from build123d import *

# Parameters (mm, degrees)
BODY_DEPTH         = 10
SKETCH2_W          = 2.5
SKETCH2_H          = 0.2
SKETCH2_W_2        = 4.5
SKETCH2_H_2        = 0.775
CUT_EXTRUDE1_DEPTH = 1.65
SKETCH3_R          = 0.757347034
WIRE_2_DEPTH       = 0.5
WIRE_2_DEPTH_BACK  = 2


with BuildPart() as part:
    # Sketch1 → Body (new body)
    with BuildSketch(Plane.XY):
        with BuildLine():
            Line((0.625, -0.775), (-0.625, -0.775))
            ThreePointArc((-0.625, -0.775), (-0.766421356, -0.716421356), (-0.825, -0.575))
            Line((-0.825, -0.575), (-0.825, 0.575))
            ThreePointArc((-0.825, 0.575), (-0.766421356, 0.716421356), (-0.625, 0.775))
            Line((-0.625, 0.775), (0.625, 0.775))
            ThreePointArc((0.625, 0.775), (0.766421356, 0.716421356), (0.825, 0.575))
            Line((0.825, 0.575), (0.825, -0.575))
            ThreePointArc((0.825, -0.575), (0.766421356, -0.716421356), (0.625, -0.775))
        make_face()
        with BuildLine():
            Line((-0.725, -0.575), (-0.725, 0.575))
            ThreePointArc((-0.725, 0.575), (-0.695710678, 0.645710678), (-0.625, 0.675))
            Line((-0.625, 0.675), (0.625, 0.675))
            ThreePointArc((0.625, 0.675), (0.695710678, 0.645710678), (0.725, 0.575))
            Line((0.725, 0.575), (0.725, -0.575))
            ThreePointArc((0.725, -0.575), (0.695710678, -0.645710678), (0.625, -0.675))
            Line((0.625, -0.675), (-0.625, -0.675))
            ThreePointArc((-0.625, -0.675), (-0.695710678, -0.645710678), (-0.725, -0.575))
        make_face(mode=Mode.SUBTRACT)
    extrude(amount=BODY_DEPTH)

    # Sketch2 → Cut-Extrude1 (cut)
    with BuildSketch(Plane.ZY.offset(0.825)):
        with Locations((2.25, 0.675)):
            Rectangle(SKETCH2_W, SKETCH2_H)
        with Locations((6.75, 0.3875)):
            Rectangle(SKETCH2_W_2, SKETCH2_H_2)
    extrude(amount=-CUT_EXTRUDE1_DEPTH, mode=Mode.SUBTRACT)

    # Sketch3 → Wire 2 (add, two sides)
    with BuildSketch(Plane.XY.offset(10)) as wire_2_sk:
        Circle(SKETCH3_R)
    extrude(amount=WIRE_2_DEPTH)
    extrude(wire_2_sk.sketch, amount=-WIRE_2_DEPTH_BACK)


solid = part.part
For this review, take the finished solid that the model builds, in its own axes (mm). Round coordinates to 2 decimals unless told otherwise and drop trailing zeros. Order: outer loops, then holes, each group sorted by start corner. A loop starts at its lowest first (then second) coordinate and runs counter-clockwise, first axis right, second up. Notation, with made-up numbers: (77, 59.25) -> (134, 59.25) arc R23 ccw to (134, 94.25) -> close; hole circle Ø5 at (-35, -19.75). An arc over 180 degrees is marked (long way). Put each result on its own line as item: value.
Q1. Add section A-A on x = 0. Write out the cut boundary in (y, z) (3 decimals).
Check result:
outline: (-0.775, 0) -> (-0.675, 0) -> (-0.675, 8) -> (0.757, 8) -> (0.757, 9) -> (0.775, 9) -> (0.775, 10) -> (0.757, 10) -> (0.757, 10.5) -> (-0.757, 10.5) -> (-0.757, 10) -> (-0.775, 10) -> close; (0.675, 0) -> (0.775, 0) -> (0.775, 1) -> (0.675, 1) -> close; (0.675, 3.5) -> (0.775, 3.5) -> (0.775, 4.5) -> (0.675, 4.5) -> close
Q2. Mouldability with a two-part tool opening along X and no side actions: class faces 1 (the flat face through (0, 0.775, 9.5)), 2 (the flat face through (0, 0, 8)) as pulls with the +X half, pulls with the -X half, needs draft (parallel to the pull), parting line crosses it, or undercut.
Check result:
face 1: needs draft
face 2: undercut
Q3. Add section D-D on z = 7. Write out the cut boundary in (x, y) (3 decimals), plus the area to 3 significant figures.
Check result:
outline: (-0.825, -0.575) arc R0.2 ccw to (-0.625, -0.775) -> (0.625, -0.775) arc R0.2 ccw to (0.825, -0.575) -> (0.825, 0) -> (0.725, 0) -> (0.725, -0.575) arc R0.1 cw to (0.625, -0.675) -> (-0.625, -0.675) arc R0.1 cw to (-0.725, -0.575) -> (-0.725, 0) -> (-0.825, 0) -> close
area: 0.287 mm2
Q4. For probe 1 along Z at (x, y) = (0.15, -0.2); probe 2 along Y at (x, z) = (0.1, 8.75) (3 decimals); probe 3 along Y at (x, z) = (0.15, 8.25) (3 decimals), list the stretches that pass through material, from the lowest coordinate up. Write a range as [from, to].
Check result:
probe 1: [8, 10.5]
probe 2: [-0.775, 0.751]
probe 3: [-0.775, 0.742]
Q5. Add section B-B on z = 4. Write out the cut boundary in (x, y) (3 decimals).
Check result:
outline: (-0.825, -0.575) arc R0.2 ccw to (-0.625, -0.775) -> (0.625, -0.775) arc R0.2 ccw to (0.825, -0.575) -> (0.825, 0.575) arc R0.2 ccw to (0.625, 0.775) -> (-0.625, 0.775) arc R0.2 ccw to (-0.825, 0.575) -> close; hole (-0.725, -0.575) arc R0.1 ccw to (-0.625, -0.675) -> (0.625, -0.675) arc R0.1 ccw to (0.725, -0.575) -> (0.725, 0.575) arc R0.1 ccw to (0.625, 0.675) -> (-0.625, 0.675) arc R0.1 ccw to (-0.725, 0.575) -> close
Q6. Add section C-C on y = -0.35. Write out the cut boundary in (x, z) (3 decimals).
Check result:
outline: (-0.825, 0) -> (-0.725, 0) -> (-0.725, 10) -> (-0.825, 10) -> close; (-0.672, 8) -> (0.672, 8) -> (0.672, 10.5) -> (-0.672, 10.5) -> close; (0.725, 0) -> (0.825, 0) -> (0.825, 10) -> (0.725, 10) -> close
